from build123d import *

# Parameters (mm, degrees)
BOSS_EXTRUDE1_DEPTH = 15.5
FILLET1_R           = 3
FILLET2_R           = 2


with BuildPart() as part:
    # Sketch1 → Boss-Extrude1 (new, symmetric)
    with BuildSketch(Plane(origin=(0, 0, 0), x_dir=(0, 0, -1), z_dir=(1, 0, 0))):
        with BuildLine():
            Line((-12.5, 57.5), (-12.5, 0))
            Line((-12.5, 0), (12.5, 0))
            Line((12.5, 0), (12.5, 57.5))
            ThreePointArc((12.5, 57.5), (0, 70), (-12.5, 57.5))
        make_face()
    extrude(amount=BOSS_EXTRUDE1_DEPTH, both=True)

    # Fillet1
    fillet1_edges = [part.edges().sort_by_distance(p)[0] for p in [
        (0, 0, -12.5),
        (0, 0, 12.5),
    ]]
    fillet(fillet1_edges, radius=FILLET1_R)

    # Fillet2
    fillet2_edges = [part.edges().sort_by_distance(p)[0] for p in [
        (-15.5, 30.25, -12.5),
        (15.5, 30.25, -12.5),
        (-15.5, 0, 0),
        (-15.5, 0.878679656, 11.621320344),
        (-15.5, 0.878679656, -11.621320344),
        (15.5, 0, 0),
        (15.5, 0.878679656, 11.621320344),
        (15.5, 0.878679656, -11.621320344),
        (15.5, 70, 0),
        (-15.5, 30.25, 12.5),
        (-15.5, 70, 0),
        (15.5, 30.25, 12.5),
    ]]
    fillet(fillet2_edges, radius=FILLET2_R)


solid = part.part
Here's how the part is built. I have some questions about the finished solid (model axes, mm). Coordinates: 2 decimals unless noted, no trailing zeros. Loops run counter-clockwise (first coordinate to the right, second up) from the corner with the lowest first, then second, coordinate; pieces in that order, holes last. Notation, with made-up numbers: (46, 4) -> (69, 4) arc R18 cw to (69, 33) -> close; hole circle Ø5 at (42.5, -12). An arc over 180 degrees is marked (long way). Use one line per item in the form item = value. Start each with the question number.
(1) Will these pins go through, and if not, where does the flat tip stop? pin 1 (3 mm diameter, centred on x = -10, z = 8.5, fed in from +Y); pin 2 (4 mm diameter, centred on x = 4.5, z = -0.5, fed in from +Y); pin 3 (4 mm diameter, centred on x = -9.5, z = 8.5, fed in from +Y).
(2) Please list where these lines run through material, in increasing order: line 1 along Y through (x, z) = (5, 5.75); line 2 along Y through (x, z) = (-3, -1.75); line 3 along Z through (x, y) = (7, 59).
(3) If we section it at A-A (x = -12.5): Please give me the cut outline in (y, z), then the cut area to 3 significant figures.
Verdict:
q1.pin_1 = 67.86
q1.pin_2 = 70
q1.pin_3 = 68.18
q2.line_1 = 0 to 68.6
q2.line_2 = 0 to 69.88
q2.line_3 = -12.41 to 12.41
q3.outline = (0, -9.5) arc R3 ccw to (3, -12.5) -> (57.5, -12.5) arc R12.5 ccw to (57.5, 12.5) -> (3, 12.5) arc R3 ccw to (0, 9.5) -> close
q3.area = 1,680 mm²
